Verification items for the finished model (mm, model axes). Round coordinates to 2 decimals unless told otherwise and drop trailing zeros. Write each loop counter-clockwise with the first axis right and the second up, starting at its lowest first coordinate (ties: lowest second). Pieces come first, ordered by that corner, then holes. Notation, with made-up numbers: M -8,-23.5 L 8,-23.5 A18 ccw 8,-17.5 Z; hole C 76,3.5 d10. An arc over 180 degrees is marked long. One line per question, with ' | ' between items.
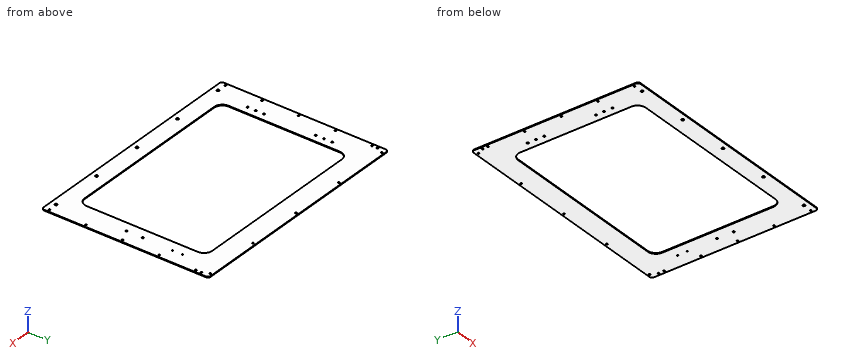
from build123d import *

# Parameters (mm, degrees)
SKETCH1_W            = 856
SKETCH1_H            = 543.9
MAINFRONT_DEPTH      = 3
SKETCH2_W            = 676
SKETCH2_H            = 463.9
DOORCUT_DEPTH        = 4
DOORROUNDINTERNAL_R  = 30
SKETCH3_W            = 856
SKETCH3_H            = 40
BOTTOMMOUNT_DEPTH    = 3
M8_CLEARANCE_HOLE1_D = 9
LPATTERN1_COUNT      = 5
LPATTERN1_PITCH      = 192.5
M5_CLEARANCE_HOLE1_D = 5.8
LPATTERN2_COUNT      = 5
LPATTERN2_PITCH      = 133.225
MIRROR1_COPY_1_D     = 5.8
MIRROR1_COPY_2_D     = 5.8
MIRROR1_COPY_3_D     = 5.8
MIRROR1_COPY_4_D     = 5.8
M5_CLEARANCE_HOLE2_D = 5.8
LPATTERN3_COUNT      = 2
LPATTERN3_PITCH      = 838
M6_CLEARANCE_HOLE1_D = 6.6
FILLET1_R            = 10
M4_CLEARANCE_HOLE1_D = 4.5
M6_CLEARANCE_HOLE2_D = 6.6
SKETCH17_W           = 856
SKETCH17_H           = 23
BOSS_EXTRUDE1_DEPTH  = 3
M5_CLEARANCE_HOLE3_D = 5.8
LPATTERN4_COUNT      = 5
LPATTERN4_PITCH      = 204
FILLET2_R            = 10


with BuildPart() as part:
    # Sketch1 → MainFront (new body)
    with BuildSketch(Plane.XY):
        with Locations((428, 271.95)):
            Rectangle(SKETCH1_W, SKETCH1_H)
    extrude(amount=MAINFRONT_DEPTH)

    # Sketch2 → DoorCut (cut, through all)
    with BuildSketch(Plane.XY.offset(3)):
        with Locations((428, 256.95)):
            Rectangle(SKETCH2_W, SKETCH2_H)
    extrude(amount=-DOORCUT_DEPTH, mode=Mode.SUBTRACT)

    # DoorRoundInternal
    doorroundinternal_edges = [part.edges().sort_by_distance(p)[0] for p in [
        (766, 488.9, 1.5),
        (766, 25, 1.5),
        (90, 25, 1.5),
        (90, 488.9, 1.5),
    ]]
    fillet(doorroundinternal_edges, radius=DOORROUNDINTERNAL_R)

    # Sketch3 → BottomMount (add)
    with BuildSketch(Plane.XY.offset(3)):
        with Locations((428, -20)):
            Rectangle(SKETCH3_W, SKETCH3_H)
    extrude(amount=-BOTTOMMOUNT_DEPTH)

    # M8 Clearance Hole1 (through all)
    with Locations(Plane.XY.offset(3)):
        with Locations((43, -20)):
            m8_clearance_hole1 = Hole(M8_CLEARANCE_HOLE1_D / 2)

    # LPattern1: M8 Clearance Hole1 ×5
    with Locations(*[(i * LPATTERN1_PITCH, 0, 0) for i in range(1, LPATTERN1_COUNT)]):
        add(m8_clearance_hole1, mode=Mode.SUBTRACT)

    # M5 Clearance Hole1 (through all)
    with Locations(Plane.XY.offset(3)):
        with Locations((9, -19)):
            m5_clearance_hole1 = Hole(M5_CLEARANCE_HOLE1_D / 2)

    # LPattern2: M5 Clearance Hole1 ×5
    with Locations(*[(0, i * LPATTERN2_PITCH, 0) for i in range(1, LPATTERN2_COUNT)]):
        add(m5_clearance_hole1, mode=Mode.SUBTRACT)

    # Mirror1: M5 Clearance Hole1 across plane
    add(m5_clearance_hole1.mirror(Plane(origin=(428, 0, 0), x_dir=(0, 0, 1), z_dir=(1, 0, 0))), mode=Mode.SUBTRACT)

    # Mirror1 copy 1 (through all)
    with Locations(Plane(origin=(856, 133.225, 3), x_dir=(-1, 0, 0), z_dir=(0, 0, 1))):
        with Locations((9, 19)):
            Hole(MIRROR1_COPY_1_D / 2)

    # Mirror1 copy 2 (through all)
    with Locations(Plane(origin=(856, 266.45, 3), x_dir=(-1, 0, 0), z_dir=(0, 0, 1))):
        with Locations((9, 19)):
            Hole(MIRROR1_COPY_2_D / 2)

    # Mirror1 copy 3 (through all)
    with Locations(Plane(origin=(856, 399.675, 3), x_dir=(-1, 0, 0), z_dir=(0, 0, 1))):
        with Locations((9, 19)):
            Hole(MIRROR1_COPY_3_D / 2)

    # Mirror1 copy 4 (through all)
    with Locations(Plane(origin=(856, 532.9, 3), x_dir=(-1, 0, 0), z_dir=(0, 0, 1))):
        with Locations((9, 19)):
            Hole(MIRROR1_COPY_4_D / 2)

    # M5 Clearance Hole2 (through all)
    with Locations(Plane.XY.offset(3)):
        with Locations((9, 533.9)):
            m5_clearance_hole2 = Hole(M5_CLEARANCE_HOLE2_D / 2)

    # LPattern3: M5 Clearance Hole2 ×2
    with Locations(*[(i * LPATTERN3_PITCH, 0, 0) for i in range(1, LPATTERN3_COUNT)]):
        add(m5_clearance_hole2, mode=Mode.SUBTRACT)

    # M6 Clearance Hole1 (through all)
    with Locations(Plane.XY.offset(3)):
        with Locations((802, 286.95), (802, 226.95)):
            Hole(M6_CLEARANCE_HOLE1_D / 2)

    # Fillet1
    fillet1_edges = [part.edges().sort_by_distance(p)[0] for p in [
        (0, -40, 1.5),
        (856, -40, 1.5),
    ]]
    fillet(fillet1_edges, radius=FILLET1_R)

    # M4 Clearance Hole1 (through all)
    with Locations(Plane.XY.offset(3)):
        with Locations((804.180642757, 432.408967428), (804.180642757, 396.408967428)):
            Hole(M4_CLEARANCE_HOLE1_D / 2)

    # M6 Clearance Hole2 (through all)
    with Locations(Plane.XY.offset(3)):
        with Locations((63, 410.9), (63, 380.9), (63, 350.9)):
            m6_clearance_hole2 = Hole(M6_CLEARANCE_HOLE2_D / 2)

    # Mirror2: M6 Clearance Hole2 across plane
    add(m6_clearance_hole2.mirror(Plane.ZX.offset(256.95)), mode=Mode.SUBTRACT)

    # Sketch17 → Boss-Extrude1 (add)
    with BuildSketch(Plane(origin=(0, 0, 0), x_dir=(-1, 0, 0), z_dir=(0, 0, -1))):
        with Locations((-428, 555.4)):
            Rectangle(SKETCH17_W, SKETCH17_H)
    extrude(amount=-BOSS_EXTRUDE1_DEPTH)

    # M5 Clearance Hole3 (through all)
    with Locations(Plane.XY.offset(3)):
        with Locations((20, 557.9)):
            m5_clearance_hole3 = Hole(M5_CLEARANCE_HOLE3_D / 2)

    # LPattern4: M5 Clearance Hole3 ×5
    with Locations(*[(i * LPATTERN4_PITCH, 0, 0) for i in range(1, LPATTERN4_COUNT)]):
        add(m5_clearance_hole3, mode=Mode.SUBTRACT)

    # Fillet2
    fillet2_edges = [part.edges().sort_by_distance(p)[0] for p in [
        (856, 566.9, 1.5),
        (0, 566.9, 1.5),
    ]]
    fillet(fillet2_edges, radius=FILLET2_R)


solid = part.part
1. Section check C-C, the plane z = 1.95. Count the separate pieces of the cut face and the enclosed holes in it, then the cut area to 3 significant figures.
Results:
separate pieces: 1 | enclosed holes: 33 | area: 206,000 mm2
2. Go/stop test with a flat-tipped pin: P1, Ø4, axis at x = 63, y = 380.9, coming from the +Z side. Record where the tip stops, or that it passes through.
Results:
P1: passes through
3. Thickness scan on line 1 (X direction, y = 163, z = 2.3); line 2 (X direction, y = 557.9, z = 1.65); line 3 (Y direction, x = 554, z = 2.45). Record the ranges inside material, lowest first.
Results:
line 1: x = 0 to 59.7, 66.3 to 90, 766 to 856 | line 2: x = 0.05 to 17.1, 22.9 to 221.1, 226.9 to 425.1, 430.9 to 629.1, 634.9 to 833.1, 838.9 to 855.95 | line 3: y = -40 to 25, 488.9 to 566.9
4. Section check A-A, the plane y = 187.5. Record the cut outline in (x, z), then the cut area to 3 significant figures.
Results:
outline: M 0,0 L 90,0 L 90,3 L 0,3 Z; M 766,0 L 856,0 L 856,3 L 766,3 Z | area: 540 mm2
5. Section check B-B, the plane x = 304. Record the cut outline in (y, z), then the cut area to 3 significant figures.
Results:
outline: M -40,0 L 25,0 L 25,3 L -40,3 Z; M 488.9,0 L 566.9,0 L 566.9,3 L 488.9,3 Z | area: 429 mm2
